Answer from the drawing. Dimensions are ordinates in mm from the lowest x, y and z of the part. A direction names the side the tool comes from. Round coordinates to 2 decimals unless told otherwise and drop trailing zeros. Order: outer loops, then holes, each group sorted by start corner. A loop starts at its lowest first (then second) coordinate and runs counter-clockwise, first axis right, second up.
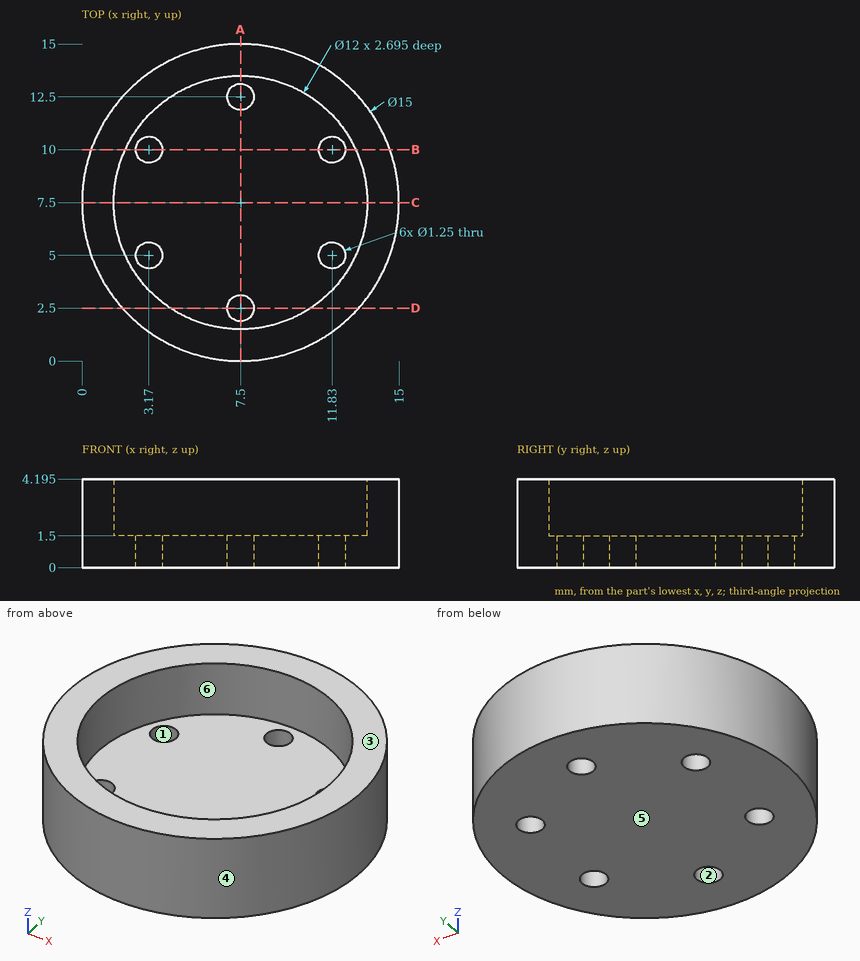
Q1. Flat-ended cylindrical pins translate along their axes: pin 1 (1.6 mm diameter, centred on x = 7.5, y = 12.5, fed in from +Z); pin 2 (1.1 mm diameter, centred on x = 11.83, y = 10, fed in from -Z). Find the tip coordinate at first contact, or state that the pin passes through.
Outcome:
pin 1: stops at z = 1.5
pin 2: passes through
Q2. A cutting plane is placed at D-D, the plane y = 2.5. Give the vertices of the cut face in (x, z) (1 decimal).
Outcome:
outline: (1.9, 0) - (6.9, 0) - (6.9, 1.5) - (4.2, 1.5) - (4.2, 4.2) - (1.9, 4.2) - close; (8.1, 0) - (13.1, 0) - (13.1, 4.2) - (10.8, 4.2) - (10.8, 1.5) - (8.1, 1.5) - close
Q3. Straight lines are drawn through the part: probe 1 along Y at (x, z) = (7.5, 1.25) (3 decimals); probe 2 along Y at (x, z) = (7.5, 1.65); probe 3 along Y at (x, z) = (11.5, 0.9). For each, find the intervals that lie inside material, in ascending order.
Outcome:
probe 1: y = 0 to 1.875, 3.125 to 11.875, 13.125 to 15
probe 2: y = 0 to 1.5, 13.5 to 15
probe 3: y = 1.16 to 4.47, 5.53 to 9.47, 10.53 to 13.84
Q4. A cutting plane is placed at C-C, the plane y = 7.5. Give the vertices of the cut face in (x, z) (3 decimals).
Outcome:
outline: (0, 0) - (15, 0) - (15, 4.195) - (13.5, 4.195) - (13.5, 1.5) - (1.5, 1.5) - (1.5, 4.195) - (0, 4.195) - close
Q5. For a pull along Y with two mould halves and no side action, classify the marked faces 1, 2, 3 and 4 as released by +Y, released by -Y, zero draft, split by the parting line, or undercut.
Outcome:
face 1: undercut
face 2: undercut
face 3: zero draft
face 4: split by the parting line
Q6. A cutting plane is placed at B-B, the plane y = 10. Give the vertices of the cut face in (x, z) (1 decimal).
Outcome:
outline: (0.4, 0) - (2.5, 0) - (2.5, 1.5) - (2, 1.5) - (2, 4.2) - (0.4, 4.2) - close; (3.8, 0) - (11.2, 0) - (11.2, 1.5) - (3.8, 1.5) - close; (12.5, 0) - (14.6, 0) - (14.6, 4.2) - (13, 4.2) - (13, 1.5) - (12.5, 1.5) - close
Q7. A cutting plane is placed at A-A, the plane x = 7.5. Give the vertices of the cut face in (y, z) (3 decimals).
Outcome:
outline: (0, 0) - (1.875, 0) - (1.875, 1.5) - (1.5, 1.5) - (1.5, 4.195) - (0, 4.195) - close; (3.125, 0) - (11.875, 0) - (11.875, 1.5) - (3.125, 1.5) - close; (13.125, 0) - (15, 0) - (15, 4.195) - (13.5, 4.195) - (13.5, 1.5) - (13.125, 1.5) - close
Q8. For the marked faces 5 and 6, determine the directions among +Z, -Z, +X, -X, +Y, -Y from which every point of the face is accessible in a straight line to the end or side of a thin tool.
Outcome:
face 5: -Z, +X, -X, +Y, -Y
face 6: +Z
